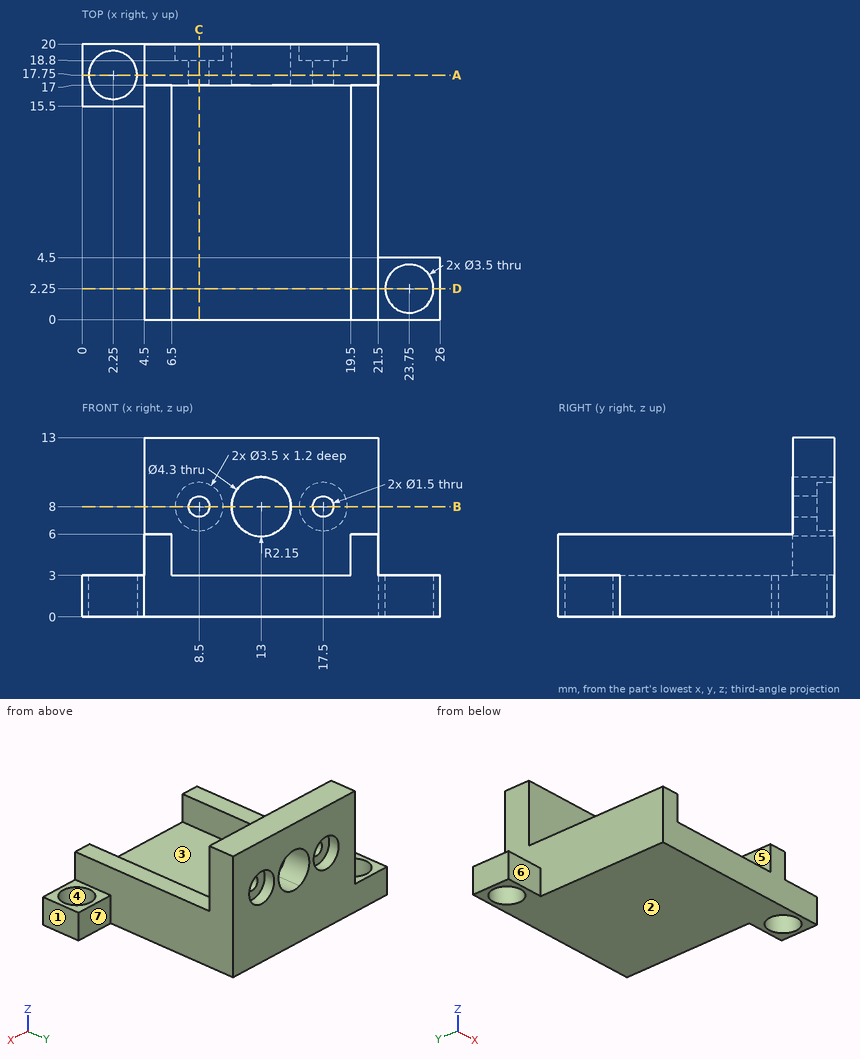
Design review of the part shown in the three views and the two pictorial views. Dimensions are in mm from the part's minimum x, y and z. A direction names the side the tool comes from. Round coordinates to 2 decimals unless told otherwise and drop trailing zeros. Loops run counter-clockwise (first coordinate to the right, second up) from the corner with the lowest first, then second, coordinate; pieces in that order, holes last. Notation, with made-up numbers: (58.5, 37.25) - (95.5, 37.25) arc R15 cw to (95.5, 43.25) - close; hole circle Ø11 at (17, -27.75). An arc over 180 degrees is marked (long way). Use CSV: the item, a comma, the result in double quotes.
(1) Take a section at D-D, the plane y = 2.25. Give the boundary of the cut face in (x, z), plus the area to 3 significant figures.
Working result:
outline,"(4.5, 0) - (22, 0) - (22, 3) - (21.5, 3) - (21.5, 6) - (19.5, 6) - (19.5, 3) - (6.5, 3) - (6.5, 6) - (4.5, 6) - close; (25.5, 0) - (26, 0) - (26, 3) - (25.5, 3) - close"
area,"66.0 mm^2"
(2) Take a section at C-C, the plane x = 8.5. Give the boundary of the cut face in (y, z).
Working result:
outline,"(0, 0) - (20, 0) - (20, 6.25) - (18.8, 6.25) - (18.8, 7.25) - (17, 7.25) - (17, 3) - (0, 3) - close; (17, 8.75) - (18.8, 8.75) - (18.8, 9.75) - (20, 9.75) - (20, 13) - (17, 13) - close"
(3) Clearance check with flat-ended pins moving along their axes: P1, Ø3.5, axis at y = 10.5, z = 5, coming from the -X side; P2, Ø1.8, axis at x = 18, z = 7.5, coming from the +Y side; P3, Ø4, axis at x = 23.75, y = 2.25, coming from the +Z side; P4, Ø7, axis at x = 13, z = 8, coming from the +Y side. State where each tip first meets the part, or that it passes through.
Working result:
P1,"stops at x = 4.5"
P2,"stops at y = 18.8"
P3,"stops at z = 3"
P4,"stops at y = 20"
(4) Machinability: for the marked faces 4, 5, 6 and 7, which of the approach directions +Z, -Z, +X, -X, +Y, -Y give a long, thin tool a straight path to every point of the face, cutting with its end or side? Answer none if there is none.
Working result:
face 4,"+Z, -Z"
face 5,"+Z, -Y"
face 6,"+Z, -Z, -X, -Y"
face 7,"+Z, -Z, +X, +Y"
(5) The part is to be moulded in two halves that separate along X. For the marked faces 1, 2 and 3, say which applies: pulls with the +X half, pulls with the -X half, needs draft (parallel to the pull), parting line crosses it, or undercut.
Working result:
face 1,"pulls with the +X half"
face 2,"needs draft"
face 3,"undercut"
(6) Take a section at A-A, the plane y = 17.75. Give the boundary of the cut face in (x, z), plus the area to 3 significant figures.
Working result:
outline,"(0, 0) - (0.5, 0) - (0.5, 3) - (0, 3) - close; (4, 0) - (21.5, 0) - (21.5, 13) - (4.5, 13) - (4.5, 3) - (4, 3) - close; hole circle Ø1.5 at (8.5, 8); hole circle Ø4.3 at (13, 8); hole circle Ø1.5 at (17.5, 8)"
area,"206 mm^2"
(7) Take a section at B-B, the plane z = 8. Give the boundary of the cut face in (x, y), plus the area to 3 significant figures.
Working result:
outline,"(4.5, 17) - (7.75, 17) - (7.75, 18.8) - (6.75, 18.8) - (6.75, 20) - (4.5, 20) - close; (9.25, 17) - (10.85, 17) - (10.85, 20) - (10.25, 20) - (10.25, 18.8) - (9.25, 18.8) - close; (15.15, 17) - (16.75, 17) - (16.75, 18.8) - (15.75, 18.8) - (15.75, 20) - (15.15, 20) - close; (18.25, 17) - (21.5, 17) - (21.5, 20) - (19.25, 20) - (19.25, 18.8) - (18.25, 18.8) - close"
area,"24.3 mm^2"
(8) For line 1 (X direction, y = 17.65, z = 8); line 2 (X direction, y = 19.65, z = 8); line 3 (Y direction, x = 23.75, z = 2.05), list the stretches that pass through material, from the lowest coordinate up.
Working result:
line 1,"x = 4.5 to 7.75, 9.25 to 10.85, 15.15 to 16.75, 18.25 to 21.5"
line 2,"x = 4.5 to 6.75, 10.25 to 10.85, 15.15 to 15.75, 19.25 to 21.5"
line 3,"y = 0 to 0.5, 4 to 4.5"
